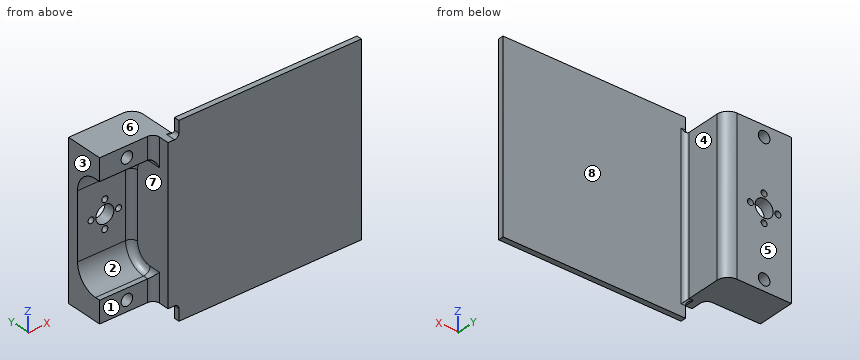
```python
from build123d import *

# Parameters (mm, degrees)
SKETCH1_W           = 106.172
SKETCH1_H           = 107.442
BOSS_EXTRUDE1_DEPTH = 3.175
SKETCH13_W          = 38.1
SKETCH13_H          = 88.9
BOSS_EXTRUDE7_DEPTH = 31.75
SKETCH15_R          = 3.3655
SKETCH15_R_2        = 5.22699996
SKETCH15_R_3        = 1.750000056
CUT_EXTRUDE1_DEPTH  = 124.152352495
SKETCH17_W          = 63.5
SKETCH17_H          = 25.4
CUT_EXTRUDE2_DEPTH  = 31.75
SKETCH18_W          = 31.75
SKETCH18_H          = 9.779
CUT_EXTRUDE3_DEPTH  = 149.047631947
FILLET2_R           = 12.7
FILLET1_R           = 3.81
FILLET3_R           = 2.54
FILLET4_R           = 2.54
FILLET5_R           = 6.35


with BuildPart() as part:
    # Sketch1 → Boss-Extrude1 (new body)
    with BuildSketch(Plane(origin=(0, 0, 0), x_dir=(1, 0, 0), z_dir=(0, 1, 0))):
        with Locations((53.086, 0)):
            Rectangle(SKETCH1_W, SKETCH1_H)
    extrude(amount=BOSS_EXTRUDE1_DEPTH)

    # Sketch13 → Boss-Extrude7 (add)
    with BuildSketch(Plane(origin=(0, 0, 0), x_dir=(1, 0, 0), z_dir=(0, 1, 0))):
        with Locations((-19.05, 0)):
            Rectangle(SKETCH13_W, SKETCH13_H)
    extrude(amount=BOSS_EXTRUDE7_DEPTH)

    # Sketch15 → Cut-Extrude1 (cut, through all)
    with BuildSketch(Plane(origin=(0, 31.75, 0), x_dir=(1, 0, 0), z_dir=(0, 1, 0))):
        with Locations(Location((-22.225, 38.1, 0), (0, 0, 270))):
            Circle(SKETCH15_R)
        with Locations(Location((-22.225, -38.1, 0), (0, 0, 270))):
            Circle(SKETCH15_R)
        with Locations(Location((-22.225, 0, 0), (0, 0, 270))):
            Circle(SKETCH15_R_2)
        with Locations(Location((-14.224999998, 0, 0), (0, 0, 270))):
            Circle(SKETCH15_R_3)
        with Locations(Location((-22.225, -8.000000002, 0), (0, 0, 270))):
            Circle(SKETCH15_R_3)
        with Locations(Location((-30.225000002, 0, 0), (0, 0, 270))):
            Circle(SKETCH15_R_3)
        with Locations(Location((-22.225, 8.000000002, 0), (0, 0, 270))):
            Circle(SKETCH15_R_3)
    extrude(amount=-CUT_EXTRUDE1_DEPTH, mode=Mode.SUBTRACT)

    # Sketch17 → Cut-Extrude2 (cut)
    with BuildSketch(Plane.ZY.offset(38.1)):
        with Locations((0, 12.7)):
            Rectangle(SKETCH17_W, SKETCH17_H)
    extrude(amount=-CUT_EXTRUDE2_DEPTH, mode=Mode.SUBTRACT)

    # Sketch18 → Cut-Extrude3 (cut, through all)
    with BuildSketch(Plane(origin=(0, 0, -44.45), x_dir=(-1, 0, 0), z_dir=(0, 0, -1))):
        with Locations((22.225, 4.8895)):
            Rectangle(SKETCH18_W, SKETCH18_H)
    extrude(amount=-CUT_EXTRUDE3_DEPTH, mode=Mode.SUBTRACT)

    # Fillet2
    fillet2_edges = [part.edges().sort_by_distance(p)[0] for p in [
        (-22.225, 25.4, -31.75),
        (-22.225, 25.4, 31.75),
    ]]
    fillet(fillet2_edges, radius=FILLET2_R)

    # Fillet1
    fillet1_edges = [part.edges().sort_by_distance(p)[0] for p in [
        (-6.35, 9.779, 38.1),
        (-6.35, 9.779, -38.1),
        (-6.35, 25.4, 0),
        (-6.35, 11.2395, 31.75),
        (-6.35, 21.680256121, -28.030256121),
        (-6.35, 21.680256121, 28.030256121),
        (-6.35, 11.2395, -31.75),
    ]]
    fillet(fillet1_edges, radius=FILLET1_R)

    # Fillet3
    fillet3_edges = [part.edges().sort_by_distance(p)[0] for p in [
        (0, 3.175, 0),
    ]]
    fillet(fillet3_edges, radius=FILLET3_R)

    # Fillet4
    fillet4_edges = [part.edges().sort_by_distance(p)[0] for p in [
        (1.27, 3.175, 44.45),
        (1.27, 3.175, -44.45),
        (0, 1.5875, 44.45),
        (0, 1.5875, -44.45),
    ]]
    fillet(fillet4_edges, radius=FILLET4_R - 0.0001)  # a hair under: the kernel refuses the full size

    # Fillet5
    fillet5_edges = [part.edges().sort_by_distance(p)[0] for p in [
        (0, 31.75, 0),
    ]]
    fillet(fillet5_edges, radius=FILLET5_R)


solid = part.part
```
Design review of the part built by this model. Coordinates are the model's own, in mm. Face numbers are marked on the shaded views. A direction names the side the tool comes from. Give positions to 0.01 mm unless a question says otherwise; leave off trailing zeros. Loops run counter-clockwise (first coordinate to the right, second up) from the corner with the lowest first, then second, coordinate; pieces in that order, holes last. Notation, with made-up numbers: M 36,-16 L 83,-16 A14 ccw 83,4 Z; hole C -9,-39.75 d7. An arc over 180 degrees is marked long. Return JSON: item names as keys, results as strings. Group by question number.
Item 1: We need section D-D (y = 7.5). Give the boundary of the cut face in (x, z).
Item 2: Insertion check: pin 1 Ø3 at (x, z) = (-14.225, 0) entering from +Y; pin 2 Ø12 at (y, z) = (22.5, 21.5) entering from +X; pin 3 Ø1.5 at (x, y) = (-23, 10.5) entering from +Z; pin 4 Ø1.5 at (x, z) = (10.5, 34) entering from +Y (3 decimals). Each pin has a flat end and moves straight along its axis. Give the tip position at first contact, or say it passes through.
Item 3: Tool access review of the marked faces 1, 2, 3, 4 and 5: name each direction out of +Z, -Z, +X, -X, +Y, -Y from which nothing blocks a thin tool from reaching the whole face with its end or side.
Item 4: We need section B-B (z = 0). Give the boundary of the cut face in (x, y) (3 decimals).
Item 5: Mouldability with a two-part tool opening along Z and no side actions: class the marked faces 6, 7 and 8 as released by +Z, released by -Z, zero draft, split by the parting line, or undercut.
Item 6: We need section C-C (y = 28). Give the number of separate pieces and of enclosed holes in the cut face, and give its area (3 significant figures).
Item 7: For probe 1 along X at (y, z) = (26, 0) (3 decimals); probe 2 along X at (y, z) = (30.5, 0) (3 decimals); probe 3 along X at (y, z) = (16, 38), list the stretches that pass through material, from the lowest coordinate up.
Output:
{
 "1": {"outline": "M -6.67,-44.45 L 0,-44.45 L 0,44.45 L -6.67,44.45 L -6.67,29.47 A3.81 cw -6.35,27.94 L -6.35,-27.94 A3.81 cw -6.67,-29.47 Z"},
 "2": {"pin 1": "passes through", "pin 2": "stops at x = 0", "pin 3": "stops at z = 44.45", "pin 4": "stops at y = 3.175"},
 "3": {"face 1": "+Z, -Z, -X, -Y", "face 2": "-X, -Y", "face 3": "+Z, -Z, -X, +Y, -Y", "face 4": "+Z, -Z, +X, +Y", "face 5": "+Z, -Z, +X, -X, +Y"},
 "4": {"outline": "M -38.1,25.4 L -31.975,25.4 L -31.975,31.75 L -38.1,31.75 Z; M -28.475,25.4 L -27.452,25.4 L -27.452,31.75 L -28.475,31.75 Z; M -16.998,25.4 L -15.975,25.4 L -15.975,31.75 L -16.998,31.75 Z; M -12.475,25.4 L -10.16,25.4 A3.81 cw -6.35,21.59 L -6.35,0 L 106.172,0 L 106.172,3.175 L 2.54,3.175 A2.54 cw 0,5.715 L 0,25.4 A6.35 ccw -6.35,31.75 L -12.475,31.75 Z"},
 "5": {"face 6": "released by +Z", "face 7": "undercut", "face 8": "zero draft"},
 "6": {"separate pieces": "1", "enclosed holes": "7", "area": "3,140 mm^2"},
 "7": {"probe 1": "x = -38.1 to -31.975, -28.475 to -27.452, -16.998 to -15.975, -12.475 to -0.028", "probe 2": "x = -38.1 to -31.975, -28.475 to -27.452, -16.998 to -15.975, -12.475 to -2.567", "probe 3": "x = -38.1 to -25.59, -18.86 to 0"}
}
